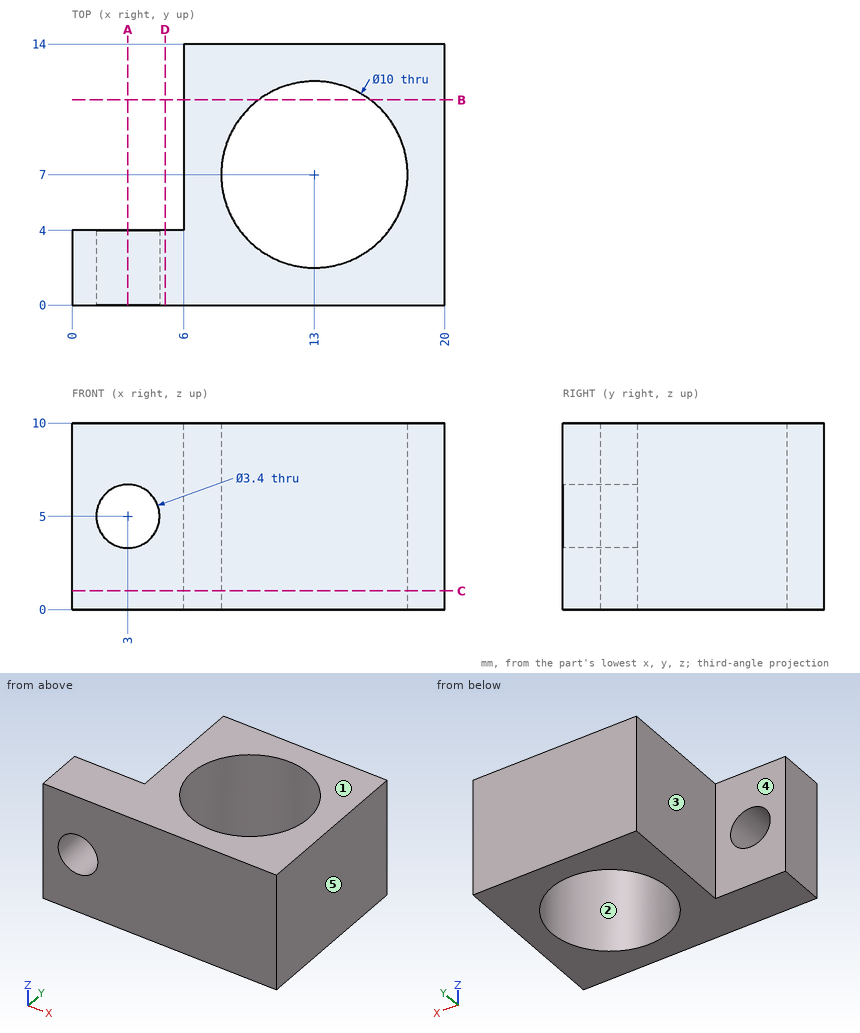
Job drawing, mm, ordinate dimensions from the low corner. One solid piece. A direction names the side the tool comes from. Coordinates: 2 decimals unless noted, no trailing zeros. Write each loop counter-clockwise with the first axis right and the second up, starting at its lowest first coordinate (ties: lowest second). Pieces come first, ordered by that corner, then holes. Notation, with made-up numbers: (72.5, 48) - (109.5, 48) arc R30 cw to (109.5, 70) - close; hole circle Ø9 at (-28, -34). An arc over 180 degrees is marked (long way). Use a Markdown table: item, result. Add a question column.
Item 1: Band-saw the part on A-A, the plane x = 3. Give the cut face in (y, z).
Item 2: Band-saw the part on D-D, the plane x = 5. Give the cut face in (y, z), and give its area (3 significant figures).
Item 3: Band-saw the part on C-C, the plane z = 1. Give the cut face in (x, y).
Item 4: Flat gauge pins, fed straight in: pin 1 (5 mm diameter, centred on x = 1.5, z = 2.5, fed in from +Y); pin 2 (4 mm diameter, centred on y = 3, z = 8, fed in from -X); pin 3 (3 mm diameter, centred on y = 8.5, z = 5.5, fed in from -X); pin 4 (8 mm diameter, centred on x = 13, y = 7, fed in from +Z). Where does each tip first touch, or does it go through?
Item 5: Drill centre lines: L1, parallel to Z at x = 3, y = 2.8; L2, parallel to Y at x = 13, z = 6; L3, parallel to X at y = 12.5, z = 0.75. Where is each one in solid material? Low to high. Write a range as from..to.
Item 6: Mould opens along X. For the marked faces 1, 2 and 3 say: pulls with the +X half, pulls with the -X half, needs draft (parallel to the pull), parting line crosses it, or undercut.
Item 7: 3-axis set-ups, long thin cutter, end or side, ignore diameter. For the marked faces 4 and 5: which of +Z, -Z, +X, -X, +Y, -Y reach the whole face in a straight line?
Item 8: Band-saw the part on B-B, the plane y = 11. Give the cut face in (x, z).
Numbers:
| question | item | result |
|---|---|---|
| 1 | outline | (0, 0) - (4, 0) - (4, 3.3) - (0, 3.3) - close; (0, 6.7) - (4, 6.7) - (4, 10) - (0, 10) - close |
| 2 | outline | (0, 0) - (4, 0) - (4, 10) - (0, 10) - close |
| 2 | area | 40.0 mm2 |
| 3 | outline | (0, 0) - (20, 0) - (20, 14) - (6, 14) - (6, 4) - (0, 4) - close; hole circle Ø10 at (13, 7) |
| 4 | pin 1 | y = 4 |
| 4 | pin 2 | x = 0 |
| 4 | pin 3 | x = 6 |
| 4 | pin 4 | through |
| 5 | L1 | 0..3.3, 6.7..10 |
| 5 | L2 | 0..2, 12..14 |
| 5 | L3 | 6..20 |
| 6 | face 1 | needs draft |
| 6 | face 2 | undercut |
| 6 | face 3 | pulls with the -X half |
| 7 | face 4 | +Z, -Z, -X, +Y |
| 7 | face 5 | +Z, -Z, +X, +Y, -Y |
| 8 | outline | (6, 0) - (10, 0) - (10, 10) - (6, 10) - close; (16, 0) - (20, 0) - (20, 10) - (16, 10) - close |
